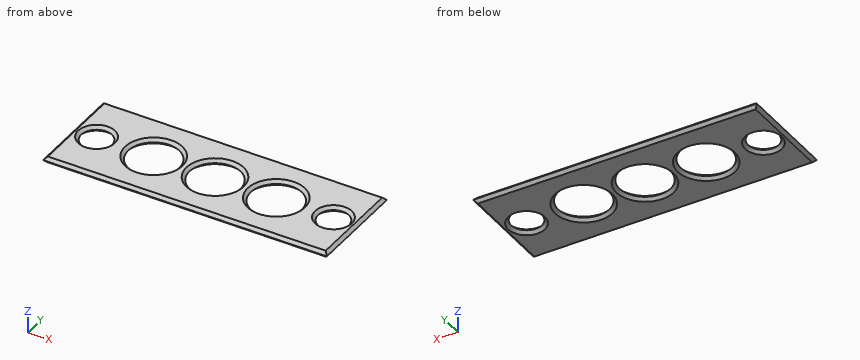
from build123d import *

# Parameters (mm, degrees)
F0_W        = 70
F0_H        = 25
F1_DEPTH    = 1.5
F2_D        = 7
F3_D        = 12
F4_SIZE     = 1
F5_T1_DEPTH = 75.1433659759
F5_T3_DEPTH = 30.1433659759


# Not quite as in the source:
# - a fillet or chamfer that OpenCascade refuses, or shapes differently, is made with other operations: its cross-section is extruded or revolved along the edge and cut away or added


with BuildPart() as f1:
    # F0 (on Top) → F1 (new body)
    with BuildSketch(Plane.XY):
        Rectangle(F0_W, F0_H)
    extrude(amount=F1_DEPTH)

    # F2 (through all)
    with Locations(Plane(origin=(0, 0, 0), x_dir=(1, 0, 0), z_dir=(0, 0, -1))):
        with Locations((-29, 0), (29, 0)):
            Hole(F2_D / 2)

    # F3 (through all)
    with Locations(Plane(origin=(0, 0, 0), x_dir=(1, 0, 0), z_dir=(0, 0, -1))):
        with Locations((-15, 0), (0, 0), (15, 0)):
            Hole(F3_D / 2)

    # F4
    f4_edges = [f1.edges().sort_by_distance(p)[0] for p in [
        (0, -12.5, 1.5),
        (-35, 0, 1.5),
        (35, 0, 1.5),
        (0, 12.5, 1.5),
        (-32.5, 0, 1.5),
        (-21, 0, 1.5),
        (-6, 0, 1.5),
        (9, 0, 1.5),
        (25.5, 0, 1.5),
    ]]
    chamfer(f4_edges, length=F4_SIZE)

    # F5: chamfer of 1 on 9 edges, made by hand

    # F5_s2 → F5_t1 (cut)
    with BuildSketch(Plane.YZ.offset(-37.571682988)):
        Polygon((-12.5, 1), (-11.5, 0), (-12.5, 0), align=None)
        Polygon((11.5, 0), (12.5, 1), (12.5, 0), align=None)
    extrude(amount=F5_T1_DEPTH, mode=Mode.SUBTRACT)

    # F5_s4 → F5_t3 (cut)
    with BuildSketch(Plane.XZ.offset(-15.071682988)):
        Polygon((-35, 1), (-34, 0), (-35, 0), align=None)
        Polygon((34, 0), (35, 1), (35, 0), align=None)
    extrude(amount=F5_T3_DEPTH, mode=Mode.SUBTRACT)

    # F5_s5 → F5_t6 (revolve, cut)
    with BuildSketch(Plane.XZ):
        Polygon((-24.5, 0), (-25.5, 1), (-25.5, 0), align=None)
    revolve(axis=Axis((-29, 0, 0), (0, 0, -1)), mode=Mode.SUBTRACT)

    # F5_s7 → F5_t8 (revolve, cut)
    with BuildSketch(Plane.XZ):
        Polygon((-8, 0), (-9, 1), (-9, 0), align=None)
    revolve(axis=Axis((-15, 0, 0), (0, 0, -1)), mode=Mode.SUBTRACT)

    # F5_s9 → F5_t10 (revolve, cut)
    with BuildSketch(Plane.XZ):
        Polygon((7, 0), (6, 1), (6, 0), align=None)
    revolve(axis=Axis((0, 0, 0), (0, 0, -1)), mode=Mode.SUBTRACT)

    # F5_s11 → F5_t12 (revolve, cut)
    with BuildSketch(Plane.XZ):
        Polygon((22, 0), (21, 1), (21, 0), align=None)
    revolve(axis=Axis((15, 0, 0), (0, 0, -1)), mode=Mode.SUBTRACT)

    # F5_s13 → F5_t14 (revolve, cut)
    with BuildSketch(Plane.XZ):
        Polygon((33.5, 0), (32.5, 1), (32.5, 0), align=None)
    revolve(axis=Axis((29, 0, 0), (0, 0, -1)), mode=Mode.SUBTRACT)


solid = f1.part
Here's how the part is built. I have some questions about the finished solid (model axes, mm). Round coordinates to 2 decimals unless told otherwise and drop trailing zeros. Write each loop counter-clockwise with the first axis right and the second up, starting at its lowest first coordinate (ties: lowest second). Pieces come first, ordered by that corner, then holes.
1. Suppose I cut it at D-D (y = 0). State how many separate pieces and enclosed holes the cut face has, and give its area (4 significant figures).
2. Suppose I cut it at B-B (z = 0.25). List the corners of the cut face in (x, y) for me, and give its area (3 significant figures).
3. I need wall thicknesses on L1, parallel to X at y = -6, z = 1.45; L2, parallel to X at y = 5, z = 0.6 (3 decimals); L3, parallel to Y at x = -29.5, z = 0.1. Which ranges of each line are inside material? Lowest first, please.
4. Suppose I cut it at A-A (x = -29). List the corners of the cut face in (y, z) for me.
5. Suppose I cut it at C-C (x = 0). List the corners of the cut face in (y, z) for me, and give its area (4 significant figures).
Answer sheet:
1. separate pieces: 6
1. enclosed holes: 0
1. area: 18.75 mm2
2. outline: (-34.25, -11.75) - (34.25, -11.75) - (34.25, 11.75) - (-34.25, 11.75) - close; hole circle Ø8.5 at (-29, 0); hole circle Ø13.5 at (-15, 0); hole circle Ø13.5 at (0, 0); hole circle Ø13.5 at (15, 0); hole circle Ø8.5 at (29, 0)
2. area: 1,070 mm2
3. L1: x = -34.05 to -18.51, -11.49 to -3.51, 3.51 to 11.49, 18.51 to 34.05
3. L2: x = -34.6 to -18.995, -11.005 to -3.995, 3.995 to 11.005, 18.995 to 34.6
3. L3: y = -11.6 to -4.37, 4.37 to 11.6
4. outline: (-12.25, 0.75) - (-11.5, 0) - (-4.5, 0) - (-3.75, 0.75) - (-4.5, 1.5) - (-11.5, 1.5) - close; (3.75, 0.75) - (4.5, 0) - (11.5, 0) - (12.25, 0.75) - (11.5, 1.5) - (4.5, 1.5) - close
5. outline: (-12.25, 0.75) - (-11.5, 0) - (-7, 0) - (-6.25, 0.75) - (-7, 1.5) - (-11.5, 1.5) - close; (6.25, 0.75) - (7, 0) - (11.5, 0) - (12.25, 0.75) - (11.5, 1.5) - (7, 1.5) - close
5. area: 15.75 mm2
